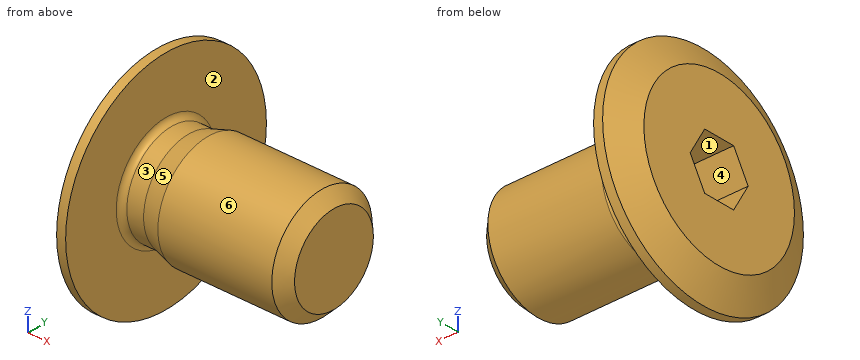
Autodesk Inventor part; units mm, degrees
ref_plane "YZ Plane" through (0, 0, 0) normal (1, 0, 0) x (0, 1, 0)
ref_plane "XZ Plane" through (0, 0, 0) normal (0, 1, 0) x (-1, 0, 0)
ref_plane "XY Plane" through (0, 0, 0) normal (0, 0, 1) x (1, 0, 0)
sketch "Sketch_1" plane through (0, 0, 0) normal (0, 0, 1) x (1, 0, 0)
  line L0 (6, 0) -> (-0.9, 0)
  line L1 (-0.9, 0) -> (-0.9, 3)
  line L2 (-0.9, 3) -> (-0.3226, 4)
  line L3 (-0.3226, 4) -> (0, 4)
  line L4 (0, 4) -> (0, 1.9852)
  arc A0 (0, 1.9852) -> (0.2, 1.7853) centre (0.2, 1.9853) ccw
  line L5 (0.2, 1.7853) -> (0.8, 1.7853)
  line L6 (0.8, 1.7853) -> (1.5, 2)
  line L7 (1.5, 2) -> (5.5705, 2)
  line L8 (5.5705, 2) -> (6, 1.5705)
  line L9 (6, 1.5705) -> (6, 0)
  line L10 (6, 0) -> (-0.9, 0)
revolve "Revolution1" add sketch "Sketch_1" angle 360 about axis through (6, 0, 0) along (1, 0, 0)
thread "Thread1"
sketch "Sketch2" plane through (-0.9, 0, 0) normal (-1, 0, 0) x (0, 0, 1)
  point P0 (0, 0)
hole "Hole1" at (-0.9, 0, 0) direction (1, 0, 0) diameter 2 depth 2.5 tip angle 120
sketch "Sketch_3" plane through (-0.9, 0, 0) normal (1, 0, 0) x (0, 0, -1)
  line L0 (-1, -0.5774) -> (0, -1.1547)
  line L1 (0, -1.1547) -> (1, -0.5774)
  line L2 (1, -0.5774) -> (1, 0.5774)
  line L3 (1, 0.5774) -> (0, 1.1547)
  line L4 (0, 1.1547) -> (-1, 0.5774)
  line L5 (-1, 0.5774) -> (-1, -0.5774)
extrude "Extrusion1" cut sketch "Sketch_3" along normal blind 2.5
properties part number "CBSTSR4-6" material "鋼、炭素鋼"
Can you work these out from the model? Positions are in its coordinate system, mm. Face numbers are marked on the shaded views. A direction names the side the tool comes from. Round coordinates to 2 decimals unless told otherwise and drop trailing zeros. Loops run counter-clockwise (first coordinate to the right, second up) from the corner with the lowest first, then second, coordinate; pieces in that order, holes last. Notation, with made-up numbers: (52.25, -14.5) -> (76.25, -14.5) arc R34 ccw to (76.25, 20.5) -> close; hole circle Ø10 at (59, -36). An arc over 180 degrees is marked (long way). Answer in a Markdown table with one row per item.
Item 1: If I drill on probe 1 along Y at (x, z) = (3, -0.25); probe 2 along X at (y, z) = (-1, 2.75); probe 3 along Y at (x, z) = (1.75, -1.75), over which ranges is the centre line in solid material (lowest first)?
Answer block:
| item | result |
|---|---|
| probe 1 | -1.98 to 1.98 |
| probe 2 | -0.9 to 0 |
| probe 3 | -0.97 to 0.97 |
Item 2: Will these pins go through, and if not, where does the flat tip stop? P1, Ø1.5, axis at x = 3.5, z = 1.5, coming from the +Y side; P2, Ø1, axis at x = 1.5, y = 1, coming from the +Z side; P3, Ø3, axis at x = 4.5, z = 3, coming from the +Y side.
Answer block:
| item | result |
|---|---|
| P1 | y = 1.85 |
| P2 | z = 1.94 |
| P3 | y = 1.32 |
Item 3: Suppose I cut it at A-A, the plane x = 2.5. List the corners of the cut face in (y, z) for me, plus the area to 3 significant figures.
Answer block:
| item | result |
|---|---|
| outline | circle Ø4 at (0, 0) |
| area | 12.6 mm² |
Item 4: We'd pull the mould along Z, two halves only. Please class the marked faces 1, 2 and 3: released by +Z, released by -Z, zero draft, split by the parting line, or undercut.
Answer block:
| item | result |
|---|---|
| face 1 | undercut |
| face 2 | zero draft |
| face 3 | split by the parting line |
Item 5: On a 3-axis mill with a long thin cutter (end or side, diameter ignored), from which of +Z, -Z, +X, -X, +Y, -Y can I reach the whole of each face in a straight line? I mean the marked faces 4, 5 and 6. Say none if no direction works.
Answer block:
| item | result |
|---|---|
| face 4 | -X |
| face 5 | none |
| face 6 | +X |
